Part print with two shaded views. Sizes in mm from the minimum x, y, z corner. Give positions to 0.01 mm unless a question says otherwise; leave off trailing zeros. Write each loop counter-clockwise with the first axis right and the second up, starting at its lowest first coordinate (ties: lowest second). Pieces come first, ordered by that corner, then holes. Notation, with made-up numbers: (55.5, 14.5) -> (67.5, 14.5) arc R17 cw to (67.5, 19.5) -> close; hole circle Ø11 at (-6.5, -40). An arc over 180 degrees is marked (long way). Write item = value, one per line. Start each with the question number.
Q1. Wall check: line 1 (Y direction, x = 3.25, z = 44.5); line 2 (X direction, y = 5.5, z = 9); line 3 (Z direction, x = 3.05, y = 7). Give the ranges that are in metal, low to high.
Q2. Mould opens along Y. For the marked faces 1 and 2 say: pulls with the +Y half, pulls with the -Y half, needs draft (parallel to the pull), parting line crosses it, or undercut.
Q3. Saw through at A-A, the plane z = 45. List the corners of the cut face in (x, y), then the cut area to 3 significant figures.
Q4. Saw through at B-B, the plane y = 12.5. List the corners of the cut face in (x, z).
Q5. Saw through at C-C, the plane y = 4. List the corners of the cut face in (x, z), then the cut area to 3 significant figures.
Q6. Saw through at D-D, the plane y = 1.25. List the corners of the cut face in (x, z), then the cut area to 3 significant figures.
Q7. Drop flat-ended pins along their axis: P1, Ø0.5, axis at x = 3.5, y = 5.5, coming from the -Z side; P2, Ø0.5, axis at x = 3.5, y = 6.5, coming from the +Z side; P3, Ø0.5, axis at x = 3.5, z = 17.5, coming from the +Y side. Give the stop position or say it passes through.
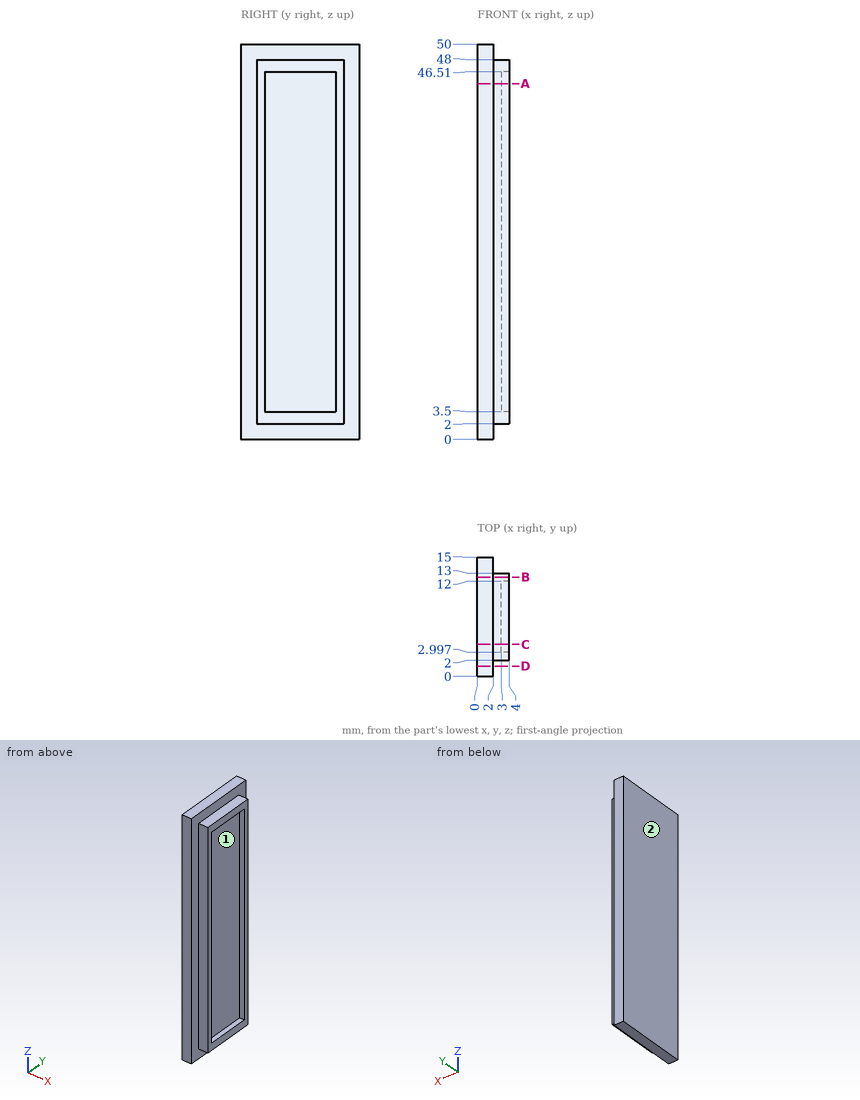
Report:
q1.line_1 = 2 to 3, 12 to 13
q1.line_2 = 0 to 3
q1.line_3 = 2 to 3.5, 46.51 to 48
q2.face_1 = undercut
q2.face_2 = needs draft
q3.outline = (0, 0) -> (2, 0) -> (2, 2) -> (4, 2) -> (4, 3) -> (3, 3) -> (3, 12) -> (4, 12) -> (4, 13) -> (2, 13) -> (2, 15) -> (0, 15) -> close
q3.area = 43.0 mm2
q4.outline = (0, 0) -> (2, 0) -> (2, 2) -> (4, 2) -> (4, 48) -> (2, 48) -> (2, 50) -> (0, 50) -> close
q5.outline = (0, 0) -> (2, 0) -> (2, 2) -> (4, 2) -> (4, 3.5) -> (3, 3.5) -> (3, 46.51) -> (4, 46.51) -> (4, 48) -> (2, 48) -> (2, 50) -> (0, 50) -> close
q5.area = 149 mm2
q6.outline = (0, 0) -> (2, 0) -> (2, 50) -> (0, 50) -> close
q6.area = 100 mm2
q7.P1 = 2
q7.P2 = 48
q7.P3 = 13
